from build123d import *

# Parameters (mm, degrees)
F0_R     = 61.10067
F1_DEPTH = 25.4
F3_D     = 12.5
F5_DEPTH = 25.4


with BuildPart() as f1:
    # F0 (on Front) → F1 (new body)
    with BuildSketch(Plane.XZ):
        Circle(F0_R)
    extrude(amount=F1_DEPTH)

    # F3 (through all)
    with Locations(Plane(origin=(0, 0, 0), x_dir=(1, 0, 0), z_dir=(0, 1, 0))):
        with Locations((0, 0)):
            Hole(F3_D / 2)

    # F4 (on face) → F5 (cut)
    with BuildSketch(Plane(origin=(0, 0, 0), x_dir=(-1, 0, 0), z_dir=(0, 1, 0))):
        with BuildLine():
            Line((-6.393978, 51.178693), (-8.104244, 51.178693))
            ThreePointArc((-8.104244, 51.178693), (0, 43.07445), (8.104244, 51.178693))
            Line((8.104244, 51.178693), (8.104244, 60.765195))
            ThreePointArc((8.104244, 60.765195), (0.855133, 68.014306), (-6.393978, 60.765195))
            Line((-6.393978, 60.765195), (-6.393978, 51.178693))
        make_face()
    extrude(amount=-F5_DEPTH, mode=Mode.SUBTRACT)


solid = f1.part
Build history of the part. All positions in model axes, mm. A direction names the side the tool comes from. Coordinates: 2 decimals unless noted, no trailing zeros. Write each loop counter-clockwise with the first axis right and the second up, starting at its lowest first coordinate (ties: lowest second). Pieces come first, ordered by that corner, then holes.
(1) Cut at A-A on z = 0. List the corners of the cut face in (x, y).
(2) Drill centre lines: line 1 (Z direction, x = 0, y = -11.5); line 2 (Z direction, x = -5.5, y = -6.75); line 3 (X direction, y = -17.25, z = -3.5). Where is each one in solid material? Low to high.
(3) Cut at D-D on x = -46.5. List the corners of the cut face in (y, z).
(4) Pin check, flat tips, straight feed: pin 1 Ø12 at (y, z) = (-19.5, -29) entering from -X; pin 2 Ø3 at (y, z) = (-16, 55) entering from -X; pin 3 Ø3 at (y, z) = (-7, 56) entering from +X; pin 4 Ø10 at (x, z) = (0, 0) entering from -Y. Stop position of each tip, or through.
(5) Mould opens along X. For faces 3 (the cylindrical face through (-1.724, -12.522, -61.076)), 4 (the cylindrical face through (-5.96, -12.88, -1.88)), 5 (the cylindrical face through (0.178, -12.522, 43.076)), 6 (the flat face through (13, -25.4, 1)) say: pulls with the +X half, pulls with the -X half, needs draft (parallel to the pull), parting line crosses it, or undercut.
(6) 3-axis set-ups, long thin cutter, end or side, ignore diameter. For faces 1 (the flat face through (6.394, -13, 56)), 2 (the flat face through (13, 0, 1)): which of +Z, -Z, +X, -X, +Y, -Y reach the whole face in a straight line?
(7) Cut at C-C on y = -16.5. List the corners of the cut face in (x, z).
(8) Cut at B-B on x = 0. List the corners of the cut face in (y, z).
Working result:
1. outline: (-61.1, -25.4) - (-6.25, -25.4) - (-6.25, 0) - (-61.1, 0) - close; (6.25, -25.4) - (61.1, -25.4) - (61.1, 0) - (6.25, 0) - close
2. line 1: z = -61.1 to -6.25, 6.25 to 43.07
2. line 2: z = -60.85 to -2.97, 2.97 to 45.23
2. line 3: x = -61 to -5.18, 5.18 to 61
3. outline: (-25.4, -39.64) - (0, -39.64) - (0, 39.64) - (-25.4, 39.64) - close
4. pin 1: stops at x = -56.61
4. pin 2: stops at x = -29.51
4. pin 3: stops at x = 27.62
4. pin 4: passes through
5. face 3: parting line crosses it
5. face 4: undercut
5. face 5: undercut
5. face 6: needs draft
6. face 1: +Z, +Y, -Y
6. face 2: +Z, -Z, +X, -X, +Y
7. outline: (-8.1, 51.18) - (-8.1, 60.56) arc R61.1 ccw (long way) to (6.39, 60.77) - (6.39, 51.18) - (8.1, 51.18) arc R8.1 cw to start; hole circle Ø12.5 at (0, 0)
8. outline: (-25.4, -61.1) - (0, -61.1) - (0, -6.25) - (-25.4, -6.25) - close; (-25.4, 6.25) - (0, 6.25) - (0, 43.07) - (-25.4, 43.07) - close
